The model under review builds one solid part; all positions refer to its coordinate system, in mm. Round coordinates to 2 decimals unless told otherwise and drop trailing zeros. Order: outer loops, then holes, each group sorted by start corner. A loop starts at its lowest first (then second) coordinate and runs counter-clockwise, first axis right, second up.
```python
from build123d import *

# Parameters (mm, degrees)
F0_W     = 109.728
F0_H     = 18.161
F1_DEPTH = 2.54
F2_R     = 3.175
F3_DEPTH = 2.541
F5_D     = 3.7973


with BuildPart() as f1:
    # F0 (on Top) → F1 (new body)
    with BuildSketch(Plane.XY):
        with Locations((54.864, 9.0805)):
            Rectangle(F0_W, F0_H)
    extrude(amount=F1_DEPTH)

    # F2 (on face) → F3 (cut, through all)
    with BuildSketch(Plane.XY.offset(2.54)):
        with Locations((9.271, 9.0805)):
            Circle(F2_R)
        with Locations((100.711, 9.0805)):
            Circle(F2_R)
    extrude(amount=-F3_DEPTH, mode=Mode.SUBTRACT)

    # F5 (through all)
    with Locations(Plane.XY.offset(2.54)):
        with Locations((29.464, 12.7), (42.0722284243, 5.08), (54.864, 12.7), (67.4722284243, 5.08), (80.264, 12.7)):
            Hole(F5_D / 2)


solid = f1.part
```
(1) To check wall thickness, follow probe 1 along X at (y, z) = (9.25, 1); probe 2 along Y at (x, z) = (80, 0.6); probe 3 along X at (y, z) = (8, 1.85). State the ranges of each line that lie inside material, in increasing order.
Data:
probe 1: x = 0 to 6.1, 12.44 to 97.54, 103.88 to 109.73
probe 2: y = 0 to 10.82, 14.58 to 18.16
probe 3: x = 0 to 6.29, 12.26 to 97.73, 103.7 to 109.73
(2) Consider section B-B (z = 1.25). State how many separate pieces and enclosed holes the cut face has, and give its area (3 significant figures).
Data:
separate pieces: 1
enclosed holes: 7
area: 1,870 mm2
(3) Consider section A-A (x = 28.5). Write out the cut boundary in (y, z).
Data:
outline: (0, 0) - (11.06, 0) - (11.06, 2.54) - (0, 2.54) - close; (14.34, 0) - (18.16, 0) - (18.16, 2.54) - (14.34, 2.54) - close
(4) Draft analysis for pull direction Y (two halves, no side actions). For faces 1 (the cylindrical face through (98.19, 7.15, 1.29)), 2 (the flat face through (54, 18.161, 1)), 3 (the flat face through (54, 0, 1)), state which applies: pulls with the +Y half, pulls with the -Y half, needs draft (parallel to the pull), parting line crosses it, or undercut.
Data:
face 1: undercut
face 2: pulls with the +Y half
face 3: pulls with the -Y half
